For this review, use the dimensioned drawing (mm, ordinates from the lowest corner) and the shaded views. Round coordinates to 2 decimals unless told otherwise and drop trailing zeros. Loops run counter-clockwise (first coordinate to the right, second up) from the corner with the lowest first, then second, coordinate; pieces in that order, holes last. Notation, with made-up numbers: (-23, -22.5) - (19, -22.5) arc R27 ccw to (19, 15.5) - close; hole circle Ø8 at (77.5, 58.25). An arc over 180 degrees is marked (long way). One line per question, with ' | ' between items. Start each with the question number.
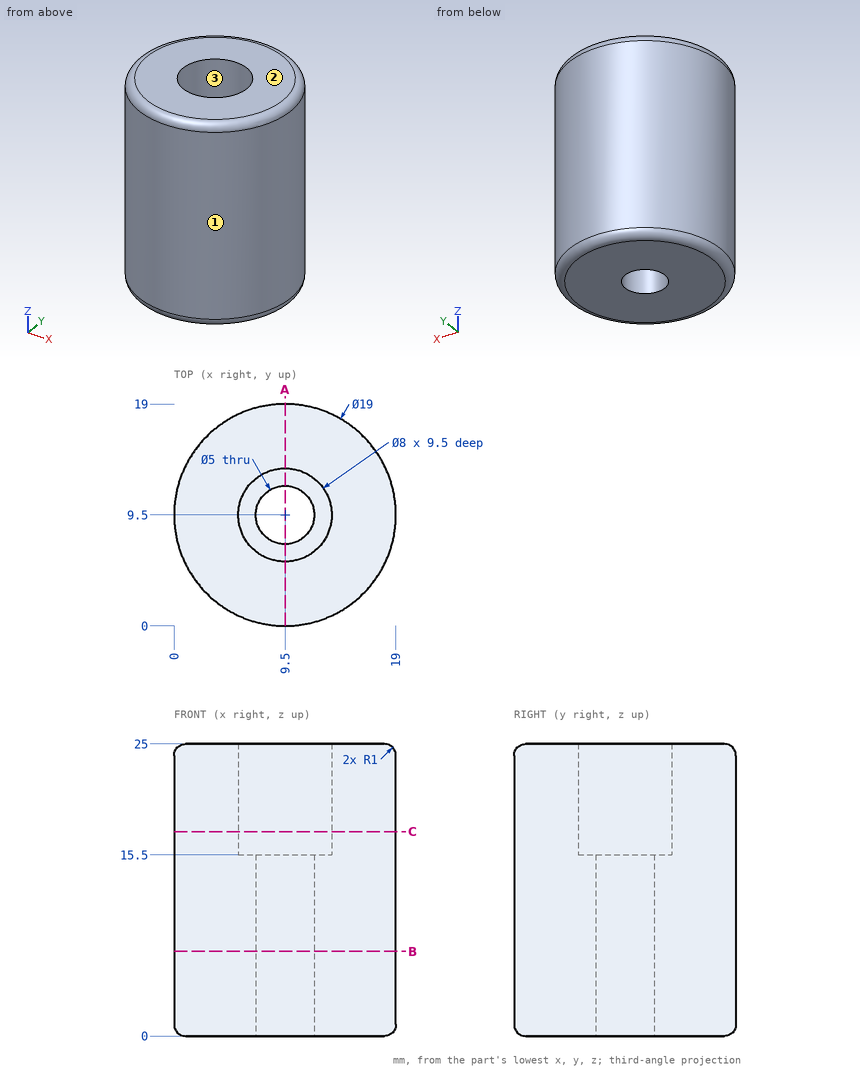
1. Take a section at C-C, the plane z = 17.5. Give the boundary of the cut face in (x, y).
2. Take a section at A-A, the plane x = 9.5. Give the boundary of the cut face in (y, z).
3. Clearance check with flat-ended pins moving along their axes: P1, Ø10, axis at x = 5, z = 8.5, coming from the +Y side; P2, Ø4, axis at y = 14.5, z = 14.5, coming from the +X side; P3, Ø3, axis at y = 16.5, z = 18.5, coming from the +X side; P4, Ø6.5, axis at x = 10, y = 10, coming from the +Z side. State where each tip first meets the part, or that it passes through.
4. To check wall thickness, follow line 1 along Y through (x, z) = (9.5, 18.25); line 2 along Y through (x, z) = (10, 9.25); line 3 along X through (y, z) = (6, 21). State the ranges of each line that lie inside material, in increasing order.
5. Take a section at B-B, the plane z = 7.25. Give the boundary of the cut face in (x, y).
6. The part is to be moulded in two halves that separate along X. For the marked faces 1, 2 and 3, say which applies: pulls with the +X half, pulls with the -X half, needs draft (parallel to the pull), parting line crosses it, or undercut.
Answer list:
1) outline: circle Ø19 at (9.5, 9.5); hole circle Ø8 at (9.5, 9.5)
2) outline: (0, 1) arc R1 ccw to (1, 0) - (7, 0) - (7, 15.5) - (5.5, 15.5) - (5.5, 25) - (1, 25) arc R1 ccw to (0, 24) - close; (12, 0) - (18, 0) arc R1 ccw to (19, 1) - (19, 24) arc R1 ccw to (18, 25) - (13.5, 25) - (13.5, 15.5) - (12, 15.5) - close
3) P1: stops at y = 19 | P2: stops at x = 18.51 | P3: stops at x = 17.25 | P4: stops at z = 15.5
4) line 1: y = 0 to 5.5, 13.5 to 19 | line 2: y = 0.01 to 7.05, 11.95 to 18.99 | line 3: x = 0.67 to 7.56, 11.44 to 18.33
5) outline: circle Ø19 at (9.5, 9.5); hole circle Ø5 at (9.5, 9.5)
6) face 1: parting line crosses it | face 2: needs draft | face 3: undercut
